```python
from build123d import *

# Parameters (mm, degrees)
SKETCH_1_W             = 39.7
SKETCH_1_H             = 85.7
EXTRUDE_1_DEPTH        = 3
SKETCH_3_W             = 10.5
SKETCH_3_H             = 10.25
SKETCH_3_H_2           = 10.5
CUT_EXTRUDE_1_DEPTH    = 3
EXTRUDE_1_2_DEPTH      = 7
EXTRUDE_1_2_DEPTH_BACK = 3
SKETCH_6_W             = 43.7
SKETCH_6_H             = 89.7
SKETCH_6_W_2           = 39.7
SKETCH_6_H_2           = 85.7
FILLET_1_R             = 6
SKETCH_7_W             = 8
SKETCH_7_H             = 3.5
CUT_EXTRUDE_2_DEPTH    = 7
FILLET_2_R             = 5
FILLET_3_R             = 5
SKETCH_8_W             = 10.5
SKETCH_8_H             = 10.5
EXTRUDE_2_DEPTH        = 3
SKETCH_9_W             = 37.1
SKETCH_9_H             = 8
CUT_EXTRUDE_3_DEPTH    = 0.6


with BuildPart() as part:
    # 스케치1 → Extrude 1 (new body)
    with BuildSketch(Plane.XY):
        Rectangle(SKETCH_1_W, SKETCH_1_H)
    extrude(amount=EXTRUDE_1_DEPTH)

    # 스케치3 → 컷-돌출1 (cut)
    with BuildSketch(Plane(origin=(0, 0, 0), x_dir=(-1, 0, 0), z_dir=(0, 0, -1))):
        with Locations((-11.3, 32.35)):
            Rectangle(SKETCH_3_W, SKETCH_3_H)
        with Locations((-11.3, 12.35)):
            Rectangle(SKETCH_3_W, SKETCH_3_H)
        with Locations((11.3, 32.35)):
            Rectangle(SKETCH_3_W, SKETCH_3_H)
        with Locations((0, 32.35)):
            Rectangle(SKETCH_3_W, SKETCH_3_H_2)
        with Locations((0, 12.35)):
            Rectangle(SKETCH_3_W, SKETCH_3_H_2)
        with Locations((11.3, 12.35)):
            Rectangle(SKETCH_3_W, SKETCH_3_H)
        with Locations((-11.3, -7.65)):
            Rectangle(SKETCH_3_W, SKETCH_3_H)
        with Locations((0, -7.65)):
            Rectangle(SKETCH_3_W, SKETCH_3_H_2)
        with Locations((11.3, -7.65)):
            Rectangle(SKETCH_3_W, SKETCH_3_H)
        with Locations((-11.3, -27.65)):
            Rectangle(SKETCH_3_W, SKETCH_3_H)
        with Locations((0, -27.65)):
            Rectangle(SKETCH_3_W, SKETCH_3_H_2)
        with Locations((11.3, -27.65)):
            Rectangle(SKETCH_3_W, SKETCH_3_H)
    extrude(amount=-CUT_EXTRUDE_1_DEPTH, mode=Mode.SUBTRACT)

    # 스케치6 → Extrude 1 2 (add, two sides: drawn at the far end of the back side and taken through both)
    with BuildSketch(Plane.XY.offset(3).offset(-EXTRUDE_1_2_DEPTH_BACK)):
        Rectangle(SKETCH_6_W, SKETCH_6_H)
        Rectangle(SKETCH_6_W_2, SKETCH_6_H_2, mode=Mode.SUBTRACT)
    extrude(amount=EXTRUDE_1_2_DEPTH + EXTRUDE_1_2_DEPTH_BACK)

    # 필렛1
    fillet_1_edges = [part.edges().sort_by_distance(p)[0] for p in [
        (21.85, 44.85, 5),
        (21.85, -44.85, 5),
        (-21.85, -44.85, 5),
        (-21.85, 44.85, 5),
    ]]
    fillet(fillet_1_edges, radius=FILLET_1_R)

    # 스케치7 → 컷-돌출2 (cut)
    with BuildSketch(Plane(origin=(0, 44.85, 0), x_dir=(1, 0, 0), z_dir=(0, 1, 0))):
        with Locations((0, -6.75)):
            Rectangle(SKETCH_7_W, SKETCH_7_H)
    extrude(amount=-CUT_EXTRUDE_2_DEPTH, mode=Mode.SUBTRACT)

    # 필렛2
    fillet_2_edges = [part.edges().sort_by_distance(p)[0] for p in [
        (-19.85, 42.85, 6.5),
        (19.85, 42.85, 6.5),
    ]]
    fillet(fillet_2_edges, radius=FILLET_2_R)

    # 필렛3
    fillet_3_edges = [part.edges().sort_by_distance(p)[0] for p in [
        (19.85, -42.85, 6.5),
        (-19.85, -42.85, 6.5),
    ]]
    fillet(fillet_3_edges, radius=FILLET_3_R)

    # 스케치8 → 보스-돌출2 (add)
    with BuildSketch(Plane(origin=(0, 0, 0), x_dir=(-1, 0, 0), z_dir=(0, 0, -1))):
        with Locations((0, 32.35)):
            Rectangle(SKETCH_8_W, SKETCH_8_H)
    extrude(amount=-EXTRUDE_2_DEPTH)

    # 스케치9 → 컷-돌출3 (cut)
    with BuildSketch(Plane(origin=(0, 0, 0), x_dir=(-1, 0, 0), z_dir=(0, 0, -1))):
        with Locations((0, 2.35)):
            Rectangle(SKETCH_9_W, SKETCH_9_H)
        with Locations((0, 22.35)):
            Rectangle(SKETCH_9_W, SKETCH_9_H)
        with Locations((0, -17.65)):
            Rectangle(SKETCH_9_W, SKETCH_9_H)
        with Locations((0, -37.65)):
            Rectangle(SKETCH_9_W, SKETCH_9_H)
    extrude(amount=-CUT_EXTRUDE_3_DEPTH, mode=Mode.SUBTRACT)


solid = part.part
```
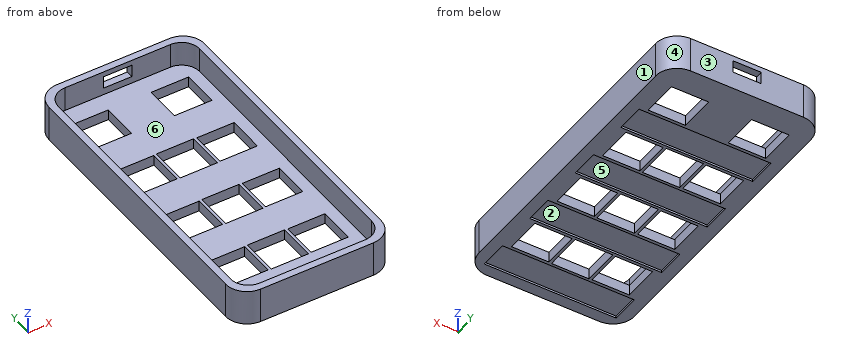
Build history of the part. All positions in model axes, mm. Face numbers are marked on the shaded views. A direction names the side the tool comes from. Coordinates: 2 decimals unless noted, no trailing zeros. Write each loop counter-clockwise with the first axis right and the second up, starting at its lowest first coordinate (ties: lowest second). Pieces come first, ordered by that corner, then holes.
1. Drop a flat-ended pin along its axis: pin 1 (4 mm diameter, centred on x = -9.5, y = -3, fed in from +Z). Give the stop position or say it passes through.
Answer block:
pin 1: stops at z = 3
2. 3-axis set-ups, long thin cutter, end or side, ignore diameter. For the marked faces 4, 5 and 6: which of +Z, -Z, +X, -X, +Y, -Y reach the whole face in a straight line?
Answer block:
face 4: +Z, -Z, +X, +Y
face 5: -Z
face 6: +Z
3. Pull direction Y, two halves, no side cores. Call the marked faces 1, 2 and 3: released by +Y, released by -Y, zero draft, split by the parting line, or undercut.
Answer block:
face 1: zero draft
face 2: undercut
face 3: released by +Y
4. Drill centre lines: probe 1 along Y at (x, z) = (-0.5, 2.25); probe 2 along X at (y, z) = (-3, 3.25); probe 3 along X at (y, z) = (29, 1). Where is each one in solid material? Low to high.
Answer block:
probe 1: y = -44.85 to -32.9, -22.4 to -12.9, -2.4 to 7.1, 17.6 to 44.85
probe 2: x = -21.85 to -19.85, 19.85 to 21.85
probe 3: x = -21.85 to -16.55, -6.05 to 6.05, 16.55 to 21.85
5. Band-saw the part on B-B, the plane y = 30. Give the cut face in (x, z).
Answer block:
outline: (-21.85, 0) - (-16.55, 0) - (-16.55, 3) - (-19.85, 3) - (-19.85, 10) - (-21.85, 10) - close; (-6.05, 0) - (6.05, 0) - (6.05, 3) - (-6.05, 3) - close; (16.55, 0) - (21.85, 0) - (21.85, 10) - (19.85, 10) - (19.85, 3) - (16.55, 3) - close
6. Band-saw the part on C-C, the plane z = 7. Give the cut face in (x, y).
Answer block:
outline: (-21.85, -38.85) arc R6 ccw to (-15.85, -44.85) - (15.85, -44.85) arc R6 ccw to (21.85, -38.85) - (21.85, 38.85) arc R6 ccw to (15.85, 44.85) - (4, 44.85) - (4, 42.85) - (14.85, 42.85) arc R5 cw to (19.85, 37.85) - (19.85, -37.85) arc R5 cw to (14.85, -42.85) - (-14.85, -42.85) arc R5 cw to (-19.85, -37.85) - (-19.85, 37.85) arc R5 cw to (-14.85, 42.85) - (-4, 42.85) - (-4, 44.85) - (-15.85, 44.85) arc R6 ccw to (-21.85, 38.85) - close
7. Band-saw the part on A-A, the plane y = -5. Give the cut face in (x, z), and give its area (3 significant figures).
Answer block:
outline: (-21.85, 0) - (-16.55, 0) - (-16.55, 3) - (-19.85, 3) - (-19.85, 10) - (-21.85, 10) - close; (-6.05, 0) - (-5.25, 0) - (-5.25, 3) - (-6.05, 3) - close; (5.25, 0) - (6.05, 0) - (6.05, 3) - (5.25, 3) - close; (16.55, 0) - (21.85, 0) - (21.85, 10) - (19.85, 10) - (19.85, 3) - (16.55, 3) - close
area: 64.6 mm2
